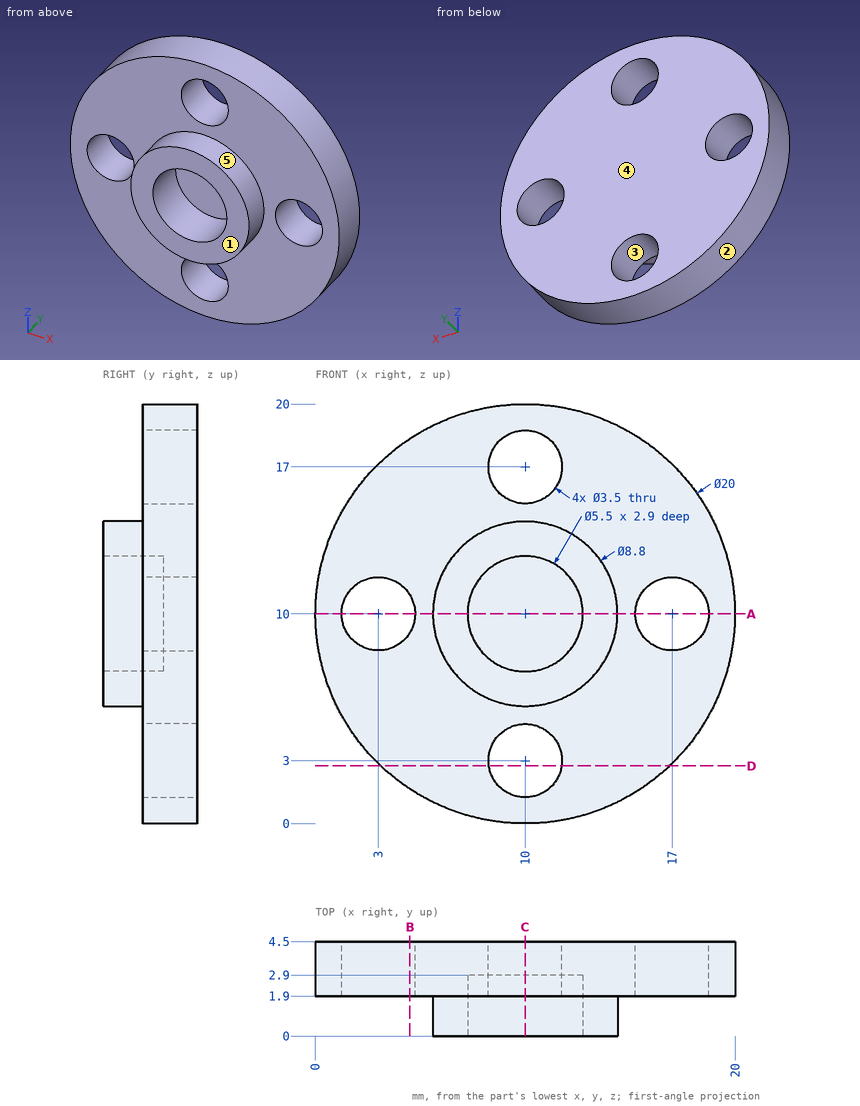
Print and shaded views of the part. All mm, measured from the part's lowest x, y and z. A direction names the side the tool comes from. Round coordinates to 2 decimals unless told otherwise and drop trailing zeros. Write each loop counter-clockwise with the first axis right and the second up, starting at its lowest first coordinate (ties: lowest second). Pieces come first, ordered by that corner, then holes. Notation, with made-up numbers: (-29, 71) -> (-24, 71) arc R10 cw to (-24, 81) -> close; hole circle Ø6 at (84.5, 69.25). An arc over 180 degrees is marked (long way). Return JSON: item names as keys, results as strings. Group by question number.
Q1. Probe L1, parallel to X at y = 2.2, z = 10; L2, parallel to Y at x = 1.75, z = 14.25; L3, parallel to X at y = 2.15, z = 18.5. List the from-to ranges inside material, lowest first. Write a range as [from, to].
Q2. Pin check, flat tips, straight feed: pin 1 (2 mm diameter, centred on y = 3, z = 8.5, fed in from -X); pin 2 (1.6 mm diameter, centred on x = 10.5, z = 10, fed in from -Y); pin 3 (4.5 mm diameter, centred on x = 10, z = 17, fed in from -Y). Stop position of each tip, or through.
Q3. Saw through at C-C on x = 10. Write the cut outline in (y, z), plus the area to 3 significant figures.
Q4. Which spindle directions (+Z, -Z, +X, -X, +Y, -Y) get a long thin tool onto all of the face, cutting with end or side? Do the marked faces 4 and 5. Say none if no direction does.
Q5. Saw through at B-B on x = 4.5. Write the cut outline in (y, z), plus the area to 3 significant figures.
Q6. Mould opens along Z. For the marked faces 1, 2 and 3 say: pulls with the +Z half, pulls with the -Z half, needs draft (parallel to the pull), parting line crosses it, or undercut.
Q7. Saw through at A-A on z = 10. Write the cut outline in (x, y).
Q8. Saw through at D-D on z = 2.75. Write the cut outline in (x, y).
Answer:
{
 "1": {"L1": "[0, 1.25], [4.75, 7.25], [12.75, 15.25], [18.75, 20]", "L2": "[1.9, 4.5]", "L3": "[4.73, 9.1], [10.9, 15.27]"},
 "2": {"pin 1": "x = 0.01", "pin 2": "y = 2.9", "pin 3": "y = 1.9"},
 "3": {"outline": "(0, 5.6) -> (1.9, 5.6) -> (1.9, 4.75) -> (4.5, 4.75) -> (4.5, 15.25) -> (1.9, 15.25) -> (1.9, 14.4) -> (0, 14.4) -> (0, 12.75) -> (2.9, 12.75) -> (2.9, 7.25) -> (0, 7.25) -> close; (1.9, 0) -> (4.5, 0) -> (4.5, 1.25) -> (1.9, 1.25) -> close; (1.9, 18.75) -> (4.5, 18.75) -> (4.5, 20) -> (1.9, 20) -> close", "area": "34.6 mm2"},
 "4": {"face 4": "+Z, -Z, +X, -X, +Y", "face 5": "-Y"},
 "5": {"outline": "(1.9, 1.65) -> (4.5, 1.65) -> (4.5, 9.1) -> (1.9, 9.1) -> close; (1.9, 10.9) -> (4.5, 10.9) -> (4.5, 18.35) -> (1.9, 18.35) -> close", "area": "38.7 mm2"},
 "6": {"face 1": "needs draft", "face 2": "parting line crosses it", "face 3": "undercut"},
 "7": {"outline": "(0, 1.9) -> (1.25, 1.9) -> (1.25, 4.5) -> (0, 4.5) -> close; (4.75, 1.9) -> (5.6, 1.9) -> (5.6, 0) -> (7.25, 0) -> (7.25, 2.9) -> (12.75, 2.9) -> (12.75, 0) -> (14.4, 0) -> (14.4, 1.9) -> (15.25, 1.9) -> (15.25, 4.5) -> (4.75, 4.5) -> close; (18.75, 1.9) -> (20, 1.9) -> (20, 4.5) -> (18.75, 4.5) -> close"},
 "8": {"outline": "(3.11, 1.9) -> (8.27, 1.9) -> (8.27, 4.5) -> (3.11, 4.5) -> close; (11.73, 1.9) -> (16.89, 1.9) -> (16.89, 4.5) -> (11.73, 4.5) -> close"}
}
